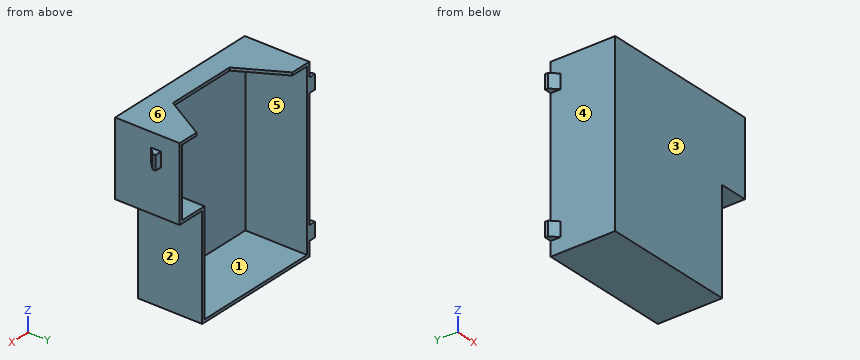
from build123d import *

# Parameters (mm, degrees)
RESSALTO_EXTRUS_O1_DEPTH  = 2
ESBO_O2_W                 = 94.5
ESBO_O2_H                 = 45.4
RESSALTO_EXTRUS_O2_DEPTH  = 2
RESSALTO_EXTRUS_O3_DEPTH  = 2
ESBO_O4_W                 = 124
ESBO_O4_H                 = 45.4
RESSALTO_EXTRUS_O4_DEPTH  = 2
ESBO_O5_W                 = 50
ESBO_O5_H                 = 45.4
RESSALTO_EXTRUS_O5_DEPTH  = 2
RESSALTO_EXTRUS_O6_START  = -10
RESSALTO_EXTRUS_O6_DEPTH  = 10
RESSALTO_EXTRUS_O7_START  = -10
RESSALTO_EXTRUS_O7_DEPTH  = 10
RESSALTO_EXTRUS_O8_START  = -10
RESSALTO_EXTRUS_O8_DEPTH  = 10
ESBO_O11_W                = 22
ESBO_O11_H                = 45.4
RESSALTO_EXTRUS_O9_DEPTH  = 2
ESBO_O14_W                = 72
ESBO_O14_H                = 45.4
RESSALTO_EXTRUS_O14_DEPTH = 2


with BuildPart() as part:
    # Esboço1 → Ressalto-extrusão1 (new body)
    with BuildSketch(Plane(origin=(0, 0, 0), x_dir=(1, 0, 0), z_dir=(0, 1, 0))):
        Polygon((57.25, -12), (37.25, -12), (37.25, 62), (-57.25, 62), (-57.25, -62), (57.25, -62), align=None)
    extrude(amount=RESSALTO_EXTRUS_O1_DEPTH)

    # Esboço2 → Ressalto-extrusão2 (add)
    with BuildSketch(Plane(origin=(0, 0, -62), x_dir=(-1, 0, 0), z_dir=(0, 0, -1))):
        with Locations((10, 22.7)):
            Rectangle(ESBO_O2_W, ESBO_O2_H)
    extrude(amount=-RESSALTO_EXTRUS_O2_DEPTH)

    # Esboço3 → Ressalto-extrusão3 (add)
    with BuildSketch(Plane.XY.offset(62)):
        Polygon((-57.25, 0), (-57.25, 45.4), (-42.25, 45.4), (-25, 15), (25, 15), (42.25, 45.4), (57.25, 45.4), (57.25, 0), align=None)
    extrude(amount=-RESSALTO_EXTRUS_O3_DEPTH)

    # Esboço4 → Ressalto-extrusão4 (add)
    with BuildSketch(Plane.ZY.offset(57.25)):
        with Locations((0, 22.7)):
            Rectangle(ESBO_O4_W, ESBO_O4_H)
    extrude(amount=-RESSALTO_EXTRUS_O4_DEPTH)

    # Esboço5 → Ressalto-extrusão5 (add)
    with BuildSketch(Plane(origin=(57.25, 0, 0), x_dir=(0, 0, -1), z_dir=(1, 0, 0))):
        with Locations((-37, 22.7)):
            Rectangle(ESBO_O5_W, ESBO_O5_H)
    extrude(amount=-RESSALTO_EXTRUS_O5_DEPTH)

    # Esboço6 → Ressalto-extrusão6 (add)
    with BuildSketch(Plane.XY.offset(62).offset(RESSALTO_EXTRUS_O6_START)):
        Polygon((57.25, 25.4), (62.199747468, 30.349747468), (62.199747468, 32.4), (57.25, 32.4), align=None)
    extrude(amount=-RESSALTO_EXTRUS_O6_DEPTH)

    # Esboço8 → Ressalto-extrusão7 (add)
    with BuildSketch(Plane.XY.offset(62).offset(RESSALTO_EXTRUS_O7_START)):
        Polygon((-57.25, 38.4), (-62.199747468, 43.349747468), (-62.199747468, 45.4), (-57.25, 45.4), align=None)
    extrude(amount=-RESSALTO_EXTRUS_O7_DEPTH)

    # Esboço10 → Ressalto-extrusão8 (add)
    with BuildSketch(Plane(origin=(0, 0, -62), x_dir=(-1, 0, 0), z_dir=(0, 0, -1)).offset(RESSALTO_EXTRUS_O8_START)):
        Polygon((57.25, 45.4), (57.25, 38.4), (62.199747468, 43.349747468), (62.199747468, 45.4), align=None)
    extrude(amount=-RESSALTO_EXTRUS_O8_DEPTH)

    # Esboço11 → Ressalto-extrusão9 (add)
    with BuildSketch(Plane(origin=(0, 0, 12), x_dir=(-1, 0, 0), z_dir=(0, 0, -1))):
        with Locations((-46.25, 22.7)):
            Rectangle(ESBO_O11_W, ESBO_O11_H)
    extrude(amount=RESSALTO_EXTRUS_O9_DEPTH)

    # Esboço14 → Ressalto-extrusão14 (add)
    with BuildSketch(Plane(origin=(37.25, 0, 0), x_dir=(0, 0, -1), z_dir=(1, 0, 0))):
        with Locations((26, 22.7)):
            Rectangle(ESBO_O14_W, ESBO_O14_H)
    extrude(amount=-RESSALTO_EXTRUS_O14_DEPTH)


solid = part.part
Input: part model. Units: mm. Frame: model coordinates. Face numbers are marked on the shaded views. A direction names the side the tool comes from. Give positions to 0.01 mm unless a question says otherwise; leave off trailing zeros. Write each loop counter-clockwise with the first axis right and the second up, starting at its lowest first coordinate (ties: lowest second). Pieces come first, ordered by that corner, then holes. Notation, with made-up numbers: M 40.5,44 L 89.5,44 A15 ccw 89.5,53 Z; hole C 27.25,1.5 d5. An arc over 180 degrees is marked long. Write item = value, one per line. Start each with the question number.
1) Material intervals for line 1 along X through (y, z) = (14.5, 9.5); line 2 along X through (y, z) = (19, 44.5); line 3 along Z through (x, y) = (46, 14.5), sorted ascending. Write a range as [from, to].
2) First-contact query: pin 1 Ø6 at (y, z) = (12, 22) entering from -X; pin 2 Ø22.5 at (y, z) = (12, 32) entering from +X; pin 3 Ø2 at (x, y) = (25, 24) entering from +Z. Flat tips, straight axial feed; report the tip coordinate or a pass-through.
3) Cut plane C-C on x = 4. Return the cut outline in (y, z).
4) Draft query along X for the marked faces 1, 2, 3 and 4. Return one class per face: +X half, -X half, draft (parallel to the pull), parting line (faces both ways), or undercut.
5) Cut plane A-A on y = 13. Return the cut outline in (x, z), then the cut area to 3 significant figures.
6) Cut plane B-B on z = 40. Return the cut outline in (x, y), then the cut area to 3 significant figures.
7) Reachability of the marked faces 5 and 6 from +Z, -Z, +X, -X, +Y, -Y: full face, straight path, thin tool, end or side. Return the list, or none.
8) Cut plane D-D on y = 41. Return the cut outline in (x, z).
Solved:
q1.line_1 = [-57.25, -55.25], [35.25, 37.25]
q1.line_2 = [-57.25, -55.25], [55.25, 57.25]
q1.line_3 = [10, 12], [60, 62]
q2.pin_1 = -57.25
q2.pin_2 = 57.25
q2.pin_3 = -60
q3.outline = M 0,-62 L 45.4,-62 L 45.4,-60 L 2,-60 L 2,60 L 15,60 L 15,62 L 0,62 Z
q4.face_1 = undercut
q4.face_2 = +X half
q4.face_3 = draft
q4.face_4 = -X half
q5.outline = M -57.25,-62 L 37.25,-62 L 37.25,10 L 57.25,10 L 57.25,62 L -57.25,62 Z; hole M -55.25,-60 L 35.25,-60 L 35.25,12 L 55.25,12 L 55.25,60 L -55.25,60 Z
q5.area = 938 mm2
q6.outline = M -57.25,0 L 57.25,0 L 57.25,45.4 L 55.25,45.4 L 55.25,2 L -55.25,2 L -55.25,45.4 L -57.25,45.4 Z
q6.area = 403 mm2
q7.face_5 = +Y
q7.face_6 = +Z, +X, -X, +Y, -Y
q8.outline = M -59.85,-52 L -57.25,-52 L -57.25,-62 L 37.25,-62 L 37.25,10 L 57.25,10 L 57.25,62 L 39.75,62 L 39.75,60 L 55.25,60 L 55.25,12 L 35.25,12 L 35.25,-60 L -55.25,-60 L -55.25,60 L -39.75,60 L -39.75,62 L -57.25,62 L -57.25,52 L -59.85,52 L -59.85,42 L -57.25,42 L -57.25,-42 L -59.85,-42 Z
